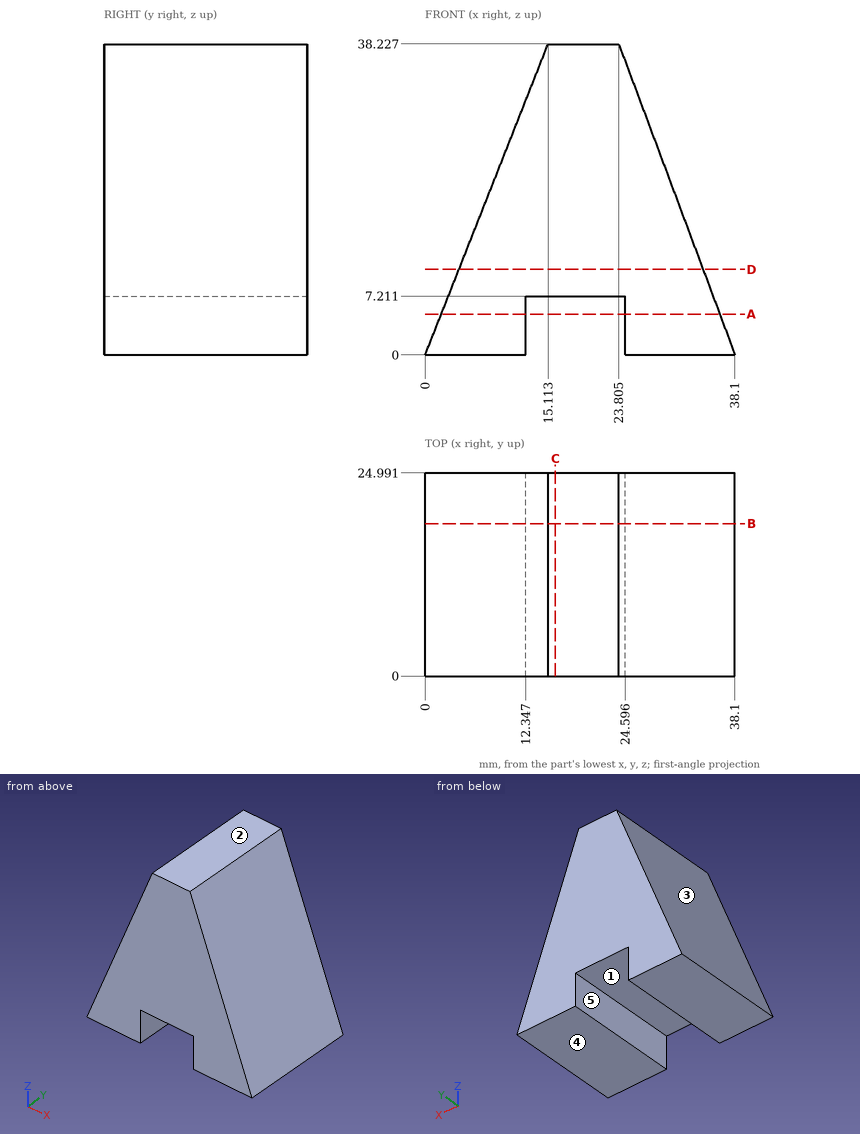
Job drawing, mm, ordinate dimensions from the low corner. One solid piece. A direction names the side the tool comes from. Give positions to 0.01 mm unless a question says otherwise; leave off trailing zeros. Order: outer loops, then holes, each group sorted by start corner. A loop starts at its lowest first (then second) coordinate and runs counter-clockwise, first axis right, second up. Notation, with made-up numbers: M 58.5,20 L 104.5,20 A15 ccw 104.5,35 Z; hole C 16,37.5 d1. An arc over 180 degrees is marked long. Return JSON: item names as keys, results as strings.
Q1. Band-saw the part on A-A (z = 5). Give the cut face in (x, y) (1 decimal).
Answer list:
{"outline": "M 2,0 L 12.3,0 L 12.3,25 L 2,25 Z; M 24.6,0 L 36.2,0 L 36.2,25 L 24.6,25 Z"}
Q2. Band-saw the part on B-B (y = 18.75). Give the cut face in (x, z) (1 decimal), then the cut area to 3 significant figures.
Answer list:
{"outline": "M 0,0 L 12.3,0 L 12.3,7.2 L 24.6,7.2 L 24.6,0 L 38.1,0 L 23.8,38.2 L 15.1,38.2 Z", "area": "806 mm^2"}
Q3. Wall check: probe 1 along Z at (x, y) = (17, 4.5); probe 2 along X at (y, z) = (18, 2) (1 decimal); probe 3 along X at (y, z) = (23.25, 4.5) (1 decimal). Give the ranges that are in metal, low to high. Write a range as from..to.
Answer list:
{"probe 1": "z = 7.21..38.23", "probe 2": "x = 0.8..12.3, 24.6..37.4", "probe 3": "x = 1.8..12.3, 24.6..36.4"}
Q4. Two-plate mould, pull along X, no slides. Class the marked faces 3, 4 and 5: pulls with the +X half, pulls with the -X half, needs draft (parallel to the pull), parting line crosses it, or undercut.
Answer list:
{"face 3": "pulls with the -X half", "face 4": "needs draft", "face 5": "undercut"}
Q5. Band-saw the part on D-D (z = 10.5). Give the cut face in (x, y).
Answer list:
{"outline": "M 4.15,0 L 34.17,0 L 34.17,24.99 L 4.15,24.99 Z"}
Q6. 3-axis set-ups, long thin cutter, end or side, ignore diameter. For the marked faces 1 and 2: which of +Z, -Z, +X, -X, +Y, -Y reach the whole face in a straight line?
Answer list:
{"face 1": "-Z, +Y, -Y", "face 2": "+Z, +X, -X, +Y, -Y"}
Q7. Flat gauge pins, fed straight in: pin 1 (2 mm diameter, centred on y = 18, z = 3, fed in from +X); pin 2 (6 mm diameter, centred on x = 30, z = 5, fed in from -Y); pin 3 (3.5 mm diameter, centred on x = 20.5, y = 16, fed in from -Z); pin 4 (3.5 mm diameter, centred on y = 11, z = 2.5, fed in from -X). Where does each tip first touch, or does it go through?
Answer list:
{"pin 1": "stops at x = 37.35", "pin 2": "stops at y = 0", "pin 3": "stops at z = 7.21", "pin 4": "stops at x = 0.3"}
Q8. Band-saw the part on C-C (x = 16). Give the cut face in (y, z), then the cut area to 3 significant figures.
Answer list:
{"outline": "M 0,7.21 L 24.99,7.21 L 24.99,38.23 L 0,38.23 Z", "area": "775 mm^2"}
